CAD build for the part. Positions are in the model's coordinates, mm. Face numbers are marked on the shaded views. A direction names the side the tool comes from. Round coordinates to 2 decimals unless told otherwise and drop trailing zeros. Loops run counter-clockwise (first coordinate to the right, second up) from the corner with the lowest first, then second, coordinate; pieces in that order, holes last. Notation, with made-up numbers: (65, 66.25) - (120, 66.25) arc R23 ccw to (120, 90.25) - close; hole circle Ø4 at (13.25, -3). An arc over 180 degrees is marked (long way). One line per question, with ' | ' between items.
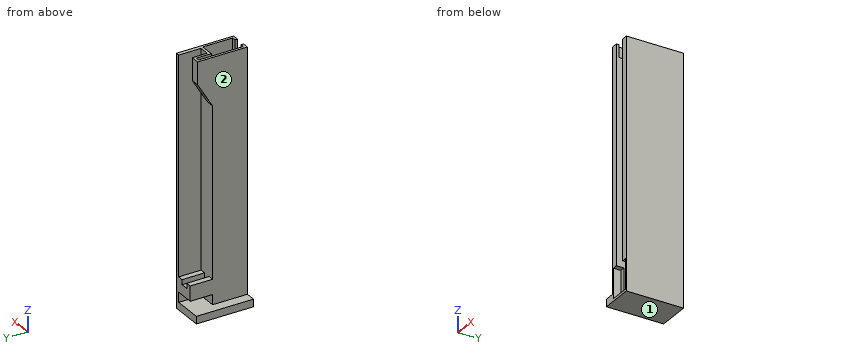
```python
from build123d import *

# Parameters (mm, degrees)
F1_DEPTH  = 23
F2_W      = 7.5
F2_H      = 4
F3_DEPTH  = 9
F5_DEPTH  = 3.5
F7_DEPTH  = 11
F9_DEPTH  = 3
F11_DEPTH = 5


with BuildPart() as f1:
    # F0 (on Front) → F1 (new body)
    with BuildSketch(Plane.XZ):
        Polygon((9, 100), (0, 100), (0, 3), (-4, 3), (-4, 0), (9, 0), align=None)
    extrude(amount=F1_DEPTH)

    # F2 (on face) → F3 (cut)
    with BuildSketch(Plane(origin=(0, 0, 0), x_dir=(-1, 0, 0), z_dir=(0, 1, 0))):
        Polygon((0, 100), (-7.5, 100), (-7.5, 13), (-5.25, 13), (-5.25, 11), (-2.25, 11), (-2.25, 13), (0, 13), align=None)
        with Locations((-3.75, 5)):
            Rectangle(F2_W, F2_H)
    extrude(amount=-F3_DEPTH, mode=Mode.SUBTRACT)

    # F4 (on face) → F5 (join)
    with BuildSketch(Plane(origin=(0, 0, 0), x_dir=(0, -1, 0), z_dir=(-1, 0, 0))):
        Polygon((9, 81), (9, 100), (3, 100), (3, 91), align=None)
    extrude(amount=-F5_DEPTH)

    # F6 (on face) → F7 (cut)
    with BuildSketch(Plane.XZ.offset(23)):
        Polygon((2.5, 100), (2.5, 97.5), (2.5, 2.5), (6.5, 2.5), (6.5, 97.5), (6.5, 100), align=None)
    extrude(amount=-F7_DEPTH, mode=Mode.SUBTRACT)

    # F8 (on face) → F9 (cut)
    with BuildSketch(Plane.XZ.offset(23)):
        Polygon((2.5, 2.5), (2.5, 13), (0.5, 13), (0.5, 1), (8.5, 1), (8.5, 13), (6.5, 13), (6.5, 2.5), align=None)
    extrude(amount=-F9_DEPTH, mode=Mode.SUBTRACT)

    # F10 (on face) → F11 (cut)
    with BuildSketch(Plane.XY.offset(100)):
        Polygon((1, -22), (2.5, -22), (2.5, -12), (6.5, -12), (6.5, -22), (8, -22), (8, -10), (2.5, -10), (2.5, -4), (1, -4), align=None)
    extrude(amount=-F11_DEPTH, mode=Mode.SUBTRACT)


solid = f1.part
```
(1) Cut at B-B, the plane z = 82. Write the cut outline in (x, y), then the cut area to 3 significant figures.
Results found:
outline: (0, -23) - (2.5, -23) - (2.5, -12) - (6.5, -12) - (6.5, -23) - (9, -23) - (9, 0) - (7.5, 0) - (7.5, -9) - (3.5, -9) - (3.5, -8.4) - (0, -8.4) - close | area: 97.6 mm²
(2) Tool access for the marked faces 1 and 2: list every direction of +Z, -Z, +X, -X, +Y, -Y with a clear straight run to the whole face (end or side of a thin tool).
Results found:
face 1: -Z, +X, -X, +Y, -Y | face 2: +Z, -X, +Y, -Y
(3) Probe L1, parallel to X at y = -17, z = 11.5; L2, parallel to Z at x = 7.75, y = -20.5; L3, parallel to Z at x = 3.5, y = -13.5. List the from-to ranges inside material, lowest first.
Results found:
L1: x = 0 to 2.5, 6.5 to 9 | L2: z = 0 to 1, 13 to 95 | L3: z = 0 to 2.5
(4) Cut at D-D, the plane x = -2.5. Write the cut outline in (y, z), then the cut area to 3 significant figures.
Results found:
outline: (-23, 0) - (0, 0) - (0, 3) - (-23, 3) - close | area: 69.0 mm²
(5) Cut at A-A, the plane y = -7.5. Write the cut outline in (x, z), then the cut area to 3 significant figures.
Results found:
outline: (-4, 0) - (9, 0) - (9, 100) - (7.5, 100) - (7.5, 13) - (5.25, 13) - (5.25, 11) - (2.25, 11) - (2.25, 13) - (0, 13) - (0, 7) - (7.5, 7) - (7.5, 3) - (-4, 3) - close; (0, 83.5) - (3.5, 83.5) - (3.5, 100) - (2.5, 100) - (2.5, 95) - (1, 95) - (1, 100) - (0, 100) - close | area: 274 mm²
(6) Cut at C-C, the plane y = -16.25. Write the cut outline in (x, z).
Results found:
outline: (-4, 0) - (9, 0) - (9, 100) - (8, 100) - (8, 95) - (6.5, 95) - (6.5, 2.5) - (2.5, 2.5) - (2.5, 95) - (1, 95) - (1, 100) - (0, 100) - (0, 3) - (-4, 3) - close
(7) Drop flat-ended pins along their axis: P1, Ø3, axis at x = 0, z = 86, coming from the +Y side; P2, Ø12, axis at y = -19.5, z = 42, coming from the -X side; P3, Ø3, axis at x = 0, z = 52.5, coming from the +Y side. Give the stop position or say it passes through.
Results found:
P1: stops at y = -5.1 | P2: stops at x = 0 | P3: stops at y = -9
